from build123d import *

# Parameters (mm, degrees)
F0_W     = 58.42
F0_H     = 93.98
F1_DEPTH = 21.082
F2_T     = -2.54
F3_W     = 13.208
F3_H     = 6.604
F4_DEPTH = 44.37549


with BuildPart() as f1:
    # F0 (on Top) → F1 (new body)
    with BuildSketch(Plane.XY):
        with Locations((8.371627, 33.384961)):
            Rectangle(F0_W, F0_H)
    extrude(amount=F1_DEPTH)

    # F2
    f2_openings = [f1.faces().sort_by_distance(p)[0] for p in [
        (8.371627, 33.384961, 21.082),
    ]]
    offset(amount=F2_T, openings=f2_openings)

    # F3 (on Front) → F4 (cut)
    with BuildSketch(Plane.XZ):
        with Locations((18.686646, 6.503384)):
            Rectangle(F3_W, F3_H)
    extrude(amount=F4_DEPTH, mode=Mode.SUBTRACT)


solid = f1.part
Work out the finished part from the listing and answer in its coordinate system (mm). A direction names the side the tool comes from. Round coordinates to 2 decimals unless told otherwise and drop trailing zeros. Write each loop counter-clockwise with the first axis right and the second up, starting at its lowest first coordinate (ties: lowest second). Pieces come first, ordered by that corner, then holes. Notation, with made-up numbers: (43.25, 85) -> (82.25, 85) arc R9 cw to (82.25, 92) -> close; hole circle Ø7 at (36, 37.25). An arc over 180 degrees is marked (long way). Answer as CSV lines item,"result". Start each with the question number.
(1) A tool of negligible diameter and unlimited length cuts with its end or side. For faces 1 (the flat face through (19, -12, 3.201)), 2 (the flat face through (8, -13.605, 10)), 3 (the flat face through (8, 77.835, 12)), from which of +Z, -Z, +X, -X, +Y, -Y can it reach the whole face along a straight path? Write none if from no direction.
(2) The mould has two halves that part along Z. Classify faces 4 (the flat face through (-20, 34, 21.082)), 5 (the flat face through (-18.298, 33, 12)), 6 (the flat face through (19, -12, 9.805)): +Z half, -Z half, draft (parallel to the pull), parting line (faces both ways), or undercut.
(3) The part is cut by section D-D, the plane x = 30.5. Give the vertices of the cut face in (y, z).
(4) Find the intervals of material crossed by probe 1 along X at (y, z) = (20, 9); probe 2 along Y at (x, z) = (2, 13.5); probe 3 along Z at (x, y) = (9, -0.5), in increasing order.
(5) The part is cut by section B-B, the plane z = 11.75. Give the vertices of the cut face in (x, y), then the cut area to 3 significant figures.
(6) The part is cut by section C-C, the plane y = 8. Give the vertices of the cut face in (x, z), then the cut area to 3 significant figures.
(7) Each of these flat-tipped pins is pushed along its axis until it touches: pin 1 (16 mm diameter, centred on x = 3.5, y = 39.5, fed in from +Z); pin 2 (5 mm diameter, centred on x = -3, y = 1.5, fed in from -Z). Where does it stop, or does it pass through?
(8) The part is cut by section A-A, the plane x = 22.5. Give the vertices of the cut face in (y, z).
Output values:
1,face 1,"-Y"
1,face 2,"+Z, -Z, +X, -X, -Y"
1,face 3,"+Z"
2,face 4,"+Z half"
2,face 5,"draft"
2,face 6,"undercut"
3,outline,"(-13.61, 0) -> (80.37, 0) -> (80.37, 21.08) -> (77.83, 21.08) -> (77.83, 2.54) -> (-11.07, 2.54) -> (-11.07, 21.08) -> (-13.61, 21.08) -> close"
4,probe 1,"x = -20.84 to -18.3, 35.04 to 37.58"
4,probe 2,"y = -13.61 to -11.07, 77.83 to 80.37"
4,probe 3,"z = 0 to 2.54"
5,outline,"(-20.84, -13.61) -> (37.58, -13.61) -> (37.58, 80.37) -> (-20.84, 80.37) -> close; hole (-18.3, -11.07) -> (35.04, -11.07) -> (35.04, 77.83) -> (-18.3, 77.83) -> close"
5,area,"748 mm²"
6,outline,"(-20.84, 0) -> (37.58, 0) -> (37.58, 21.08) -> (35.04, 21.08) -> (35.04, 2.54) -> (-18.3, 2.54) -> (-18.3, 21.08) -> (-20.84, 21.08) -> close"
6,area,"243 mm²"
7,pin 1,"stops at z = 2.54"
7,pin 2,"stops at z = 0"
8,outline,"(-13.61, 0) -> (80.37, 0) -> (80.37, 21.08) -> (77.83, 21.08) -> (77.83, 2.54) -> (-11.07, 2.54) -> (-11.07, 3.2) -> (-13.61, 3.2) -> close; (-13.61, 9.81) -> (-11.07, 9.81) -> (-11.07, 21.08) -> (-13.61, 21.08) -> close"
